Verification items for the finished model (mm, model axes). A direction names the side the tool comes from. Coordinates: 2 decimals unless noted, no trailing zeros. Loops run counter-clockwise (first coordinate to the right, second up) from the corner with the lowest first, then second, coordinate; pieces in that order, holes last.
Q1. Access from +Z, -Z, +X, -X, +Y, -Y to the whole of each face (thin tool, end or side, straight path). Record for faces 5 (the face through (9.48, -5.58, 6.9)), 6 (the face through (-2, -7, 3)).
Q2. Sectioned sample at C-C (y = 6.5). Enter the section's corners in (x, z), then the cut area to 3 significant figures.
Q3. Sectioned sample at A-A (x = 0). Enter the section's corners in (y, z), then the cut area to 3 significant figures.
Q4. Material ranges on probe 1 along Y at (x, z) = (0, 2); probe 2 along Y at (x, z) = (0, 5.5); probe 3 along Z at (x, y) = (-3.25, 7.25), recorded low to high.
Q5. Mould release check, pull along Y, two halves, no side actions. Record for faces 1 (the face through (-0.9, 6.84, 1.52)), 2 (the face through (0, -11, 7)), 3 (the face through (7.62, -3.16, 8.58)), 4 (the face through (8, 3, 14)): +Y half, -Y half, draft (parallel to the pull), parting line (faces both ways), or undercut.
Q6. Sectioned sample at B-B (z = 2.5). Enter the section's corners in (x, y), then the cut area to 3 significant figures.
Q7. Go/stop test with a flat-tipped pin: P1, Ø4, axis at y = 0, z = 5, coming from the -X side. Record where the tip stops, or that it passes through.
Q8. Sectioned sample at D-D (z = 13). Enter the section's corners in (x, y).
```python
from build123d import *

# Parameters (mm, degrees)
LINEAR_AUSTRAGEN1_DEPTH         = 14
SKIZZE2_R                       = 6.9
SCHNITT_LINEAR_AUSTRAGEN1_DEPTH = 22.870832936
SKIZZE3_R                       = 8.25
SCHNITT_LINEAR_AUSTRAGEN2_DEPTH = 11


with BuildPart() as part:
    # Skizze1 → Linear austragen1 (new body)
    with BuildSketch(Plane.XY):
        Polygon((-12.701705922, 0), (-6.350852961, -11), (6.350852961, -11), (12.701705922, 0), (6.350852961, 11), (-6.350852961, 11), align=None)
    extrude(amount=LINEAR_AUSTRAGEN1_DEPTH)

    # Skizze2 → Schnitt-Linear austragen1 (cut, through all)
    with BuildSketch(Plane.XY.offset(14)):
        Circle(SKIZZE2_R)
    extrude(amount=-SCHNITT_LINEAR_AUSTRAGEN1_DEPTH, mode=Mode.SUBTRACT)

    # Skizze3 → Schnitt-Linear austragen2 (cut)
    with BuildSketch(Plane.XY.offset(14)):
        Circle(SKIZZE3_R)
    extrude(amount=-SCHNITT_LINEAR_AUSTRAGEN2_DEPTH, mode=Mode.SUBTRACT)


solid = part.part
```
Geometry check:
1. face 5: +Z, -Z, +X, -Y
1. face 6: +Z
2. outline: (-8.95, 0) - (-2.32, 0) - (-2.32, 3) - (-5.08, 3) - (-5.08, 14) - (-8.95, 14) - close; (2.32, 0) - (8.95, 0) - (8.95, 14) - (5.08, 14) - (5.08, 3) - (2.32, 3) - close
2. area: 125 mm2
3. outline: (-11, 0) - (-6.9, 0) - (-6.9, 3) - (-8.25, 3) - (-8.25, 14) - (-11, 14) - close; (6.9, 0) - (11, 0) - (11, 14) - (8.25, 14) - (8.25, 3) - (6.9, 3) - close
3. area: 85.1 mm2
4. probe 1: y = -11 to -6.9, 6.9 to 11
4. probe 2: y = -11 to -8.25, 8.25 to 11
4. probe 3: z = 0 to 3
5. face 1: undercut
5. face 2: -Y half
5. face 3: undercut
5. face 4: draft
6. outline: (-12.7, 0) - (-6.35, -11) - (6.35, -11) - (12.7, 0) - (6.35, 11) - (-6.35, 11) - close; hole circle Ø13.8 at (0, 0)
6. area: 270 mm2
7. P1: stops at x = -12.7
8. outline: (-12.7, 0) - (-6.35, -11) - (6.35, -11) - (12.7, 0) - (6.35, 11) - (-6.35, 11) - close; hole circle Ø16.5 at (0, 0)
